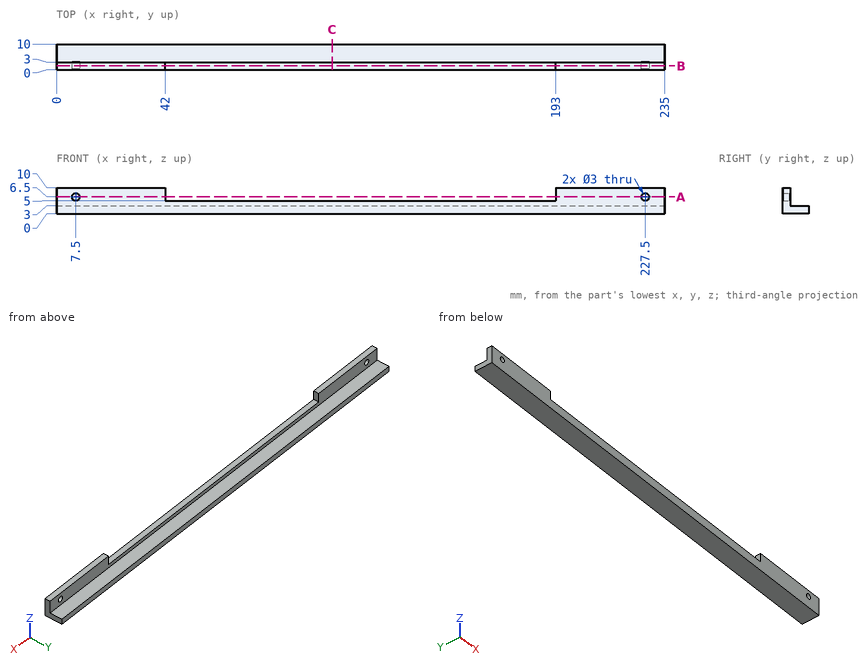
Design review of the part shown in the three views and the two pictorial views. Dimensions are in mm from the part's minimum x, y and z. Round coordinates to 2 decimals unless told otherwise and drop trailing zeros. Write each loop counter-clockwise with the first axis right and the second up, starting at its lowest first coordinate (ties: lowest second). Pieces come first, ordered by that corner, then holes. Notation, with made-up numbers: (16, 55.25) - (44, 55.25) arc R31 ccw to (44, 86.25) - close; hole circle Ø10 at (29.25, -6.5). An arc over 180 degrees is marked (long way). Answer as CSV lines item,"result". Start each with the question number.
(1) Add section C-C, the plane x = 106.5. State the section outline as (y, z) points.
(2) For line 1 (X direction, y = 0.7, z = 6.5); line 2 (Z direction, x = 7.5, y = 0.7); line 3 (X direction, y = 1.25, z = 7.25), list the stretches that pass through material, from the lowest coordinate up.
(3) Add section A-A, the plane z = 6.5. State the section outline as (x, y) points.
(4) Add section B-B, the plane y = 1.5. State the section outline as (x, z) points, plus the area to 3 significant figures.
(5) For pin 1 (1.5 mm diameter, centred on x = 172, z = 7.5, fed in from -Y); pin 2 (5.5 mm diameter, centred on x = 62.5, z = 6, fed in from +Y); pin 3 (2.5 mm diameter, centred on x = 104, y = 2, fed in from +Z); pin 4 (3.5 mm diameter, centred on x = 106, y = 6, fed in from +Z), all flat-tipped, find the tip position at first contact; note any pin that passes through.
From the geometry:
1,outline,"(0, 0) - (10, 0) - (10, 3) - (3, 3) - (3, 5) - (0, 5) - close"
2,line 1,"x = 0 to 6, 9 to 42, 193 to 226, 229 to 235"
2,line 2,"z = 0 to 5, 8 to 10"
2,line 3,"x = 0 to 6.2, 8.8 to 42, 193 to 226.2, 228.8 to 235"
3,outline,"(0, 0) - (6, 0) - (6, 3) - (0, 3) - close; (9, 0) - (42, 0) - (42, 3) - (9, 3) - close; (193, 0) - (226, 0) - (226, 3) - (193, 3) - close; (229, 0) - (235, 0) - (235, 3) - (229, 3) - close"
4,outline,"(0, 0) - (235, 0) - (235, 10) - (193, 10) - (193, 5) - (42, 5) - (42, 10) - (0, 10) - close; hole circle Ø3 at (7.5, 6.5); hole circle Ø3 at (227.5, 6.5)"
4,area,"1,580 mm²"
5,pin 1,"passes through"
5,pin 2,"stops at y = 3"
5,pin 3,"stops at z = 5"
5,pin 4,"stops at z = 3"
